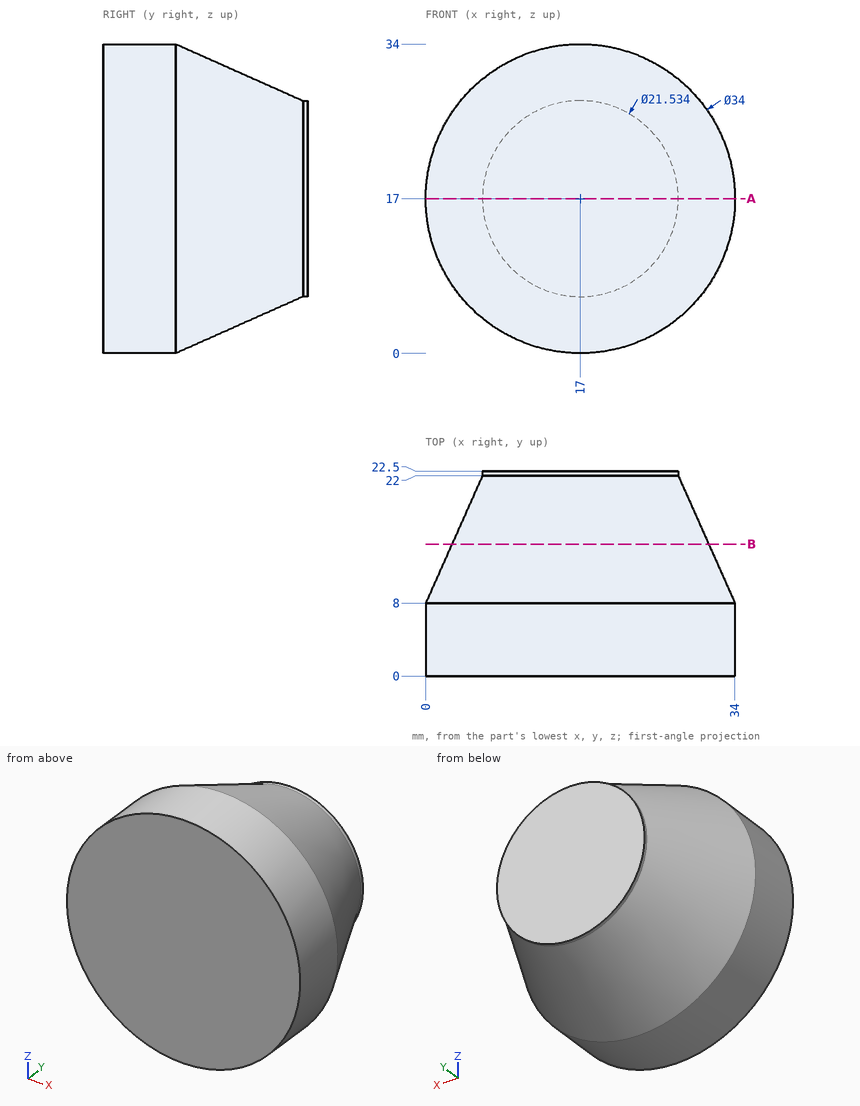
Drawing for the job (mm, zero at the part's lowest x, y, z). Give positions to 0.01 mm unless a question says otherwise; leave off trailing zeros. Loops run counter-clockwise (first coordinate to the right, second up) from the corner with the lowest first, then second, coordinate; pieces in that order, holes last. Notation, with made-up numbers: (55, 34.25) - (113, 34.25) arc R8 cw to (113, 46.25) - close; hole circle Ø1 at (74, 67). An arc over 180 degrees is marked (long way). Write item = value, one per line. Start each with the question number.
1) Band-saw the part on B-B on y = 14.5. Give the cut face in (x, z).
2) Band-saw the part on A-A on z = 17. Give the cut face in (x, y).
3) Probe probe 1 along X at (y, z) = (2, 24); probe 2 along Z at (x, y) = (27.5, 7.75); probe 3 along Y at (x, z) = (23, 2) (1 decimal). List the from-to ranges inside material, lowest first. Write a range as from..to.
4) Drop flat-ended pins along their axis: pin 1 Ø5 at (y, z) = (17.5, 18) entering from -X; pin 2 Ø12 at (y, z) = (19, 4.5) entering from +X; pin 3 Ø2 at (x, y) = (17, 17.5) entering from -Z (1 decimal). Give the stop position or say it passes through.
Final values:
q1.outline = circle Ø28.21 at (17, 17)
q2.outline = (0, 0) - (34, 0) - (34, 8) - (27.77, 22) - (27.77, 22.5) - (6.23, 22.5) - (6.23, 22) - (0, 8) - close
q3.probe_1 = 1.51..32.49
q3.probe_2 = 3.63..30.37
q3.probe_3 = 0..9.9
q4.pin_1 = 3.14
q4.pin_2 = 28.34
q4.pin_3 = 3.8
